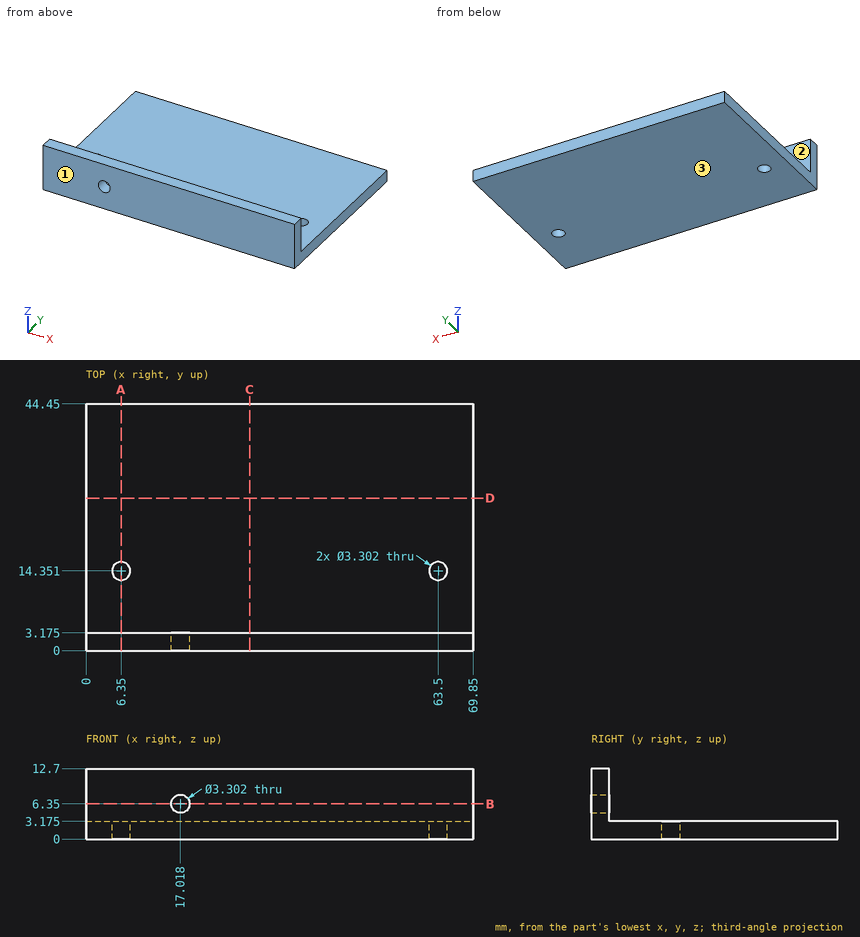
The drawing under review shows one solid part. Ordinate dimensions are in mm from its lowest x, y, z. Round coordinates to 2 decimals unless told otherwise and drop trailing zeros. Write each loop counter-clockwise with the first axis right and the second up, starting at its lowest first coordinate (ties: lowest second). Pieces come first, ordered by that corner, then holes.
(1) We need section B-B on z = 6.35. Give the boundary of the cut face in (x, y) (3 decimals), and give its area (3 significant figures).
(2) We need section A-A on x = 6.35. Give the boundary of the cut face in (y, z) (3 decimals).
(3) Mouldability with a two-part tool opening along Y and no side actions: class the marked faces 1, 2 and 3 as +Y half, -Y half, draft (parallel to the pull), parting line (faces both ways), or undercut.
(4) Wall thickness on L1, parallel to Y at x = 6.35, z = 2; L2, parallel to Z at x = 54, y = 29 (3 decimals): over which ranges is each line inside the solid? List them lowest first.
(5) We need section C-C on x = 29.5. Give the boundary of the cut face in (y, z) (3 decimals), and give its area (3 significant figures).
(6) We need section D-D on y = 27.5. Give the boundary of the cut face in (x, z) (3 decimals), and give its area (3 significant figures).
(7) Insertion check: pin 1 (4 mm diameter, centred on x = 6.35, y = 14.351, fed in from -Z); pin 2 (2 mm diameter, centred on x = 17.018, z = 6.35, fed in from +Y); pin 3 (12.5 mm diameter, centred on x = 47, y = 28, fed in from +Z) (3 decimals); pin 4 (3 mm diameter, centred on x = 32.5, z = 8.5, fed in from +Y) (3 decimals). Each pin has a flat end and moves straight along its axis. Give the tip position at first contact, or say it passes through.
Findings below:
1. outline: (0, 0) - (15.367, 0) - (15.367, 3.175) - (0, 3.175) - close; (18.669, 0) - (69.85, 0) - (69.85, 3.175) - (18.669, 3.175) - close
1. area: 211 mm2
2. outline: (0, 0) - (12.7, 0) - (12.7, 3.175) - (3.175, 3.175) - (3.175, 12.7) - (0, 12.7) - close; (16.002, 0) - (44.45, 0) - (44.45, 3.175) - (16.002, 3.175) - close
3. face 1: -Y half
3. face 2: +Y half
3. face 3: draft
4. L1: y = 0 to 12.7, 16 to 44.45
4. L2: z = 0 to 3.175
5. outline: (0, 0) - (44.45, 0) - (44.45, 3.175) - (3.175, 3.175) - (3.175, 12.7) - (0, 12.7) - close
5. area: 171 mm2
6. outline: (0, 0) - (69.85, 0) - (69.85, 3.175) - (0, 3.175) - close
6. area: 222 mm2
7. pin 1: stops at z = 0
7. pin 2: passes through
7. pin 3: stops at z = 3.175
7. pin 4: stops at y = 3.175
